Read the model definition and answer for the solid it produces. Units are mm, in the model's axes. Coordinates: 2 decimals unless noted, no trailing zeros. Order: outer loops, then holes, each group sorted by start corner. A loop starts at its lowest first (then second) coordinate and runs counter-clockwise, first axis right, second up. Notation, with made-up numbers: (25.5, 55.5) -> (61.5, 55.5) arc R22 ccw to (61.5, 94.5) -> close; hole circle Ø5 at (-39, 71.25). An arc over 180 degrees is marked (long way). Answer in a Markdown table with one row per item.
from build123d import *

# Parameters (mm, degrees)
SKETCH2_R                       = 76.1746
SKETCH2_R_2                     = 73.914
BOSS_EXTRUDE1_DEPTH             = 381
F_1_8_0_1250_DOWEL_HOLE1_REACH  = 419.341
F_1_8_0_1250_DOWEL_HOLE1_BORE_R = 1.5875
CIRPATTERN1_COUNT               = 10


with BuildPart() as part:
    # Sketch2 → Boss-Extrude1 (new body)
    with BuildSketch(Plane(origin=(0, 0, 0), x_dir=(1, 0, 0), z_dir=(0, 1, 0))):
        with Locations(Location((0, 0, 0), (0, 0, 270))):
            Circle(SKETCH2_R)
        with Locations(Location((0, 0, 0), (0, 0, 270))):
            Circle(SKETCH2_R_2, mode=Mode.SUBTRACT)
    extrude(amount=BOSS_EXTRUDE1_DEPTH)

    # 1/8 (0.1250) Dowel Hole1 bore → 1/8 (0.1250) Dowel Hole1 (cut, up to next)
    with BuildSketch(Plane(origin=(76.1746, 0, 0), x_dir=(0, 0, -1), z_dir=(1, 0, 0)), mode=Mode.PRIVATE) as f_1_8_0_1250_dowel_hole1_sk1:
        with Locations((0, 46.99)):
            Circle(F_1_8_0_1250_DOWEL_HOLE1_BORE_R)
    f_1_8_0_1250_dowel_hole1_tool1 = extrude(f_1_8_0_1250_dowel_hole1_sk1.sketch, amount=-F_1_8_0_1250_DOWEL_HOLE1_REACH, mode=Mode.PRIVATE) & part.part
    f_1_8_0_1250_dowel_hole1 = f_1_8_0_1250_dowel_hole1_tool1.solids().sort_by_distance((76.1746, 46.99, 0))[0]
    add(f_1_8_0_1250_dowel_hole1, mode=Mode.SUBTRACT)

    # CirPattern1: 1/8 (0.1250) Dowel Hole1 ×10 about axis
    cirpattern1_axis = Axis((0, 381, 0), (0, -1, 0))
    for i in range(1, CIRPATTERN1_COUNT):
        add(f_1_8_0_1250_dowel_hole1.rotate(cirpattern1_axis, i * 360 / CIRPATTERN1_COUNT), mode=Mode.SUBTRACT)


solid = part.part
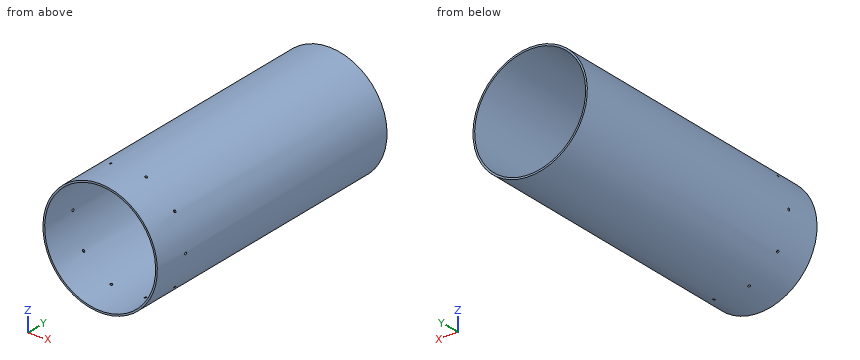
Q1. The part is cut by section B-B (z = 61). Write down the section's boundary in (x, y).
Outcome:
| item | result |
|---|---|
| outline | (-45.62, 0) -> (-41.74, 0) -> (-41.74, 381) -> (-45.62, 381) -> close; (41.74, 0) -> (45.62, 0) -> (45.62, 381) -> (41.74, 381) -> close |
Q2. Given pin 1 (3.5 mm diameter, centred on y = 46.99, z = 0, fed in from +X); pin 2 (4 mm diameter, centred on x = 22, y = 315, fed in from +Z); pin 3 (3 mm diameter, centred on x = -37, y = 199.5, fed in from -Z); pin 4 (8 mm diameter, centred on x = -60, y = 87.5, fed in from -Z), each flat-ended and moving along its own axis, determine where each tip first touches the part or whether it passes through.
Outcome:
| item | result |
|---|---|
| pin 1 | x = 76.17 |
| pin 2 | z = 73.5 |
| pin 3 | z = -67.4 |
| pin 4 | z = -51.64 |
Q3. The part is cut by section C-C (y = 284). Write down the section's boundary in (x, z), then the cut area to 3 significant figures.
Outcome:
| item | result |
|---|---|
| outline | circle Ø152.35 at (0, 0); hole circle Ø147.83 at (0, 0) |
| area | 1,070 mm² |
Q4. The part is cut by section A-A (x = 0). Write down the section's boundary in (y, z).
Outcome:
| item | result |
|---|---|
| outline | (0, -76.17) -> (381, -76.17) -> (381, -73.91) -> (0, -73.91) -> close; (0, 73.91) -> (381, 73.91) -> (381, 76.17) -> (0, 76.17) -> close |
Q5. Consider line 1 (X direction, y = 104, z = 0); line 2 (Y direction, x = 74, z = 0); line 3 (X direction, y = 352, z = 45.5). Determine where each line is inside the solid, lowest interval first.
Outcome:
| item | result |
|---|---|
| line 1 | -76.17 to -73.91, 73.91 to 76.17 |
| line 2 | 0 to 45.4, 48.58 to 381 |
| line 3 | -61.09 to -58.25, 58.25 to 61.09 |
